Could you check a few things on this drawing? It's one solid part, dimensions in mm from its lowest x, y, z. Round coordinates to 2 decimals unless told otherwise and drop trailing zeros. Order: outer loops, then holes, each group sorted by start corner. A loop starts at its lowest first (then second) coordinate and runs counter-clockwise, first axis right, second up. Notation, with made-up numbers: (49.25, 44.25) - (94.25, 44.25) arc R26 ccw to (94.25, 70.25) - close; hole circle Ø9 at (-9, 69). An arc over 180 degrees is marked (long way). Use one line per item in the form item = value.
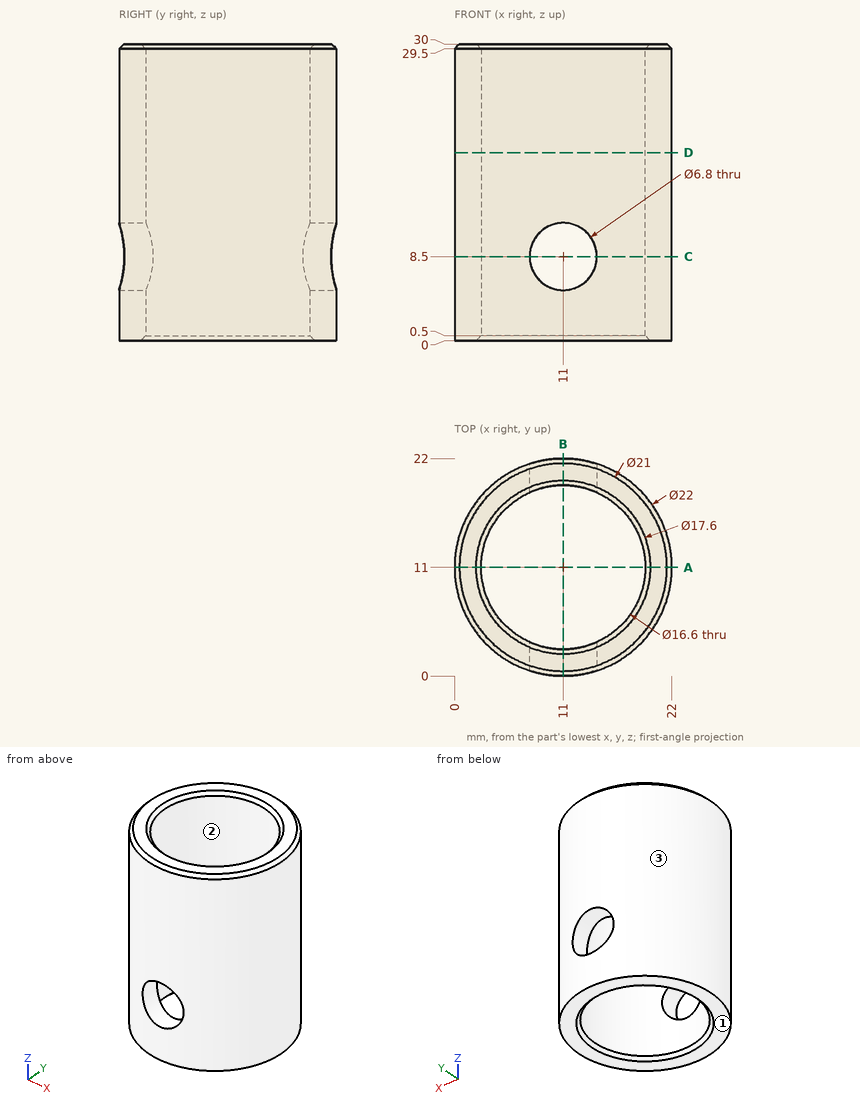
Item 1: I need wall thicknesses on L1, parallel to X at y = 10.75, z = 10; L2, parallel to Z at x = 9.25, y = 19.75. Which ranges of each line are inside material? Lowest first, please.
Found:
L1 = 0 to 2.7, 19.3 to 22
L2 = 0 to 5.58, 11.42 to 30
Item 2: Will these pins go through, and if not, where does the flat tip stop? P1, Ø12, axis at x = 17, y = 13, coming from the +Z side; P2, Ø5.5, axis at x = 11, z = 8.5, coming from the +Y side; P3, Ø1, axis at x = 3.5, z = 9, coming from the -Y side; P4, Ø6, axis at y = 3, z = 14.5, coming from the +X side.
Found:
P1 = 30
P2 = through
P3 = 2.51
P4 = 20.8
Item 3: Imagine slicing it at B-B on x = 11. Please give me the cut outline in (y, z).
Found:
outline = (0, 0) - (2.2, 0) - (2.7, 0.5) - (2.7, 5.1) - (0, 5.1) - close; (0, 11.9) - (2.7, 11.9) - (2.7, 29.5) - (2.2, 30) - (0.5, 30) - (0, 29.5) - close; (19.3, 0.5) - (19.8, 0) - (22, 0) - (22, 5.1) - (19.3, 5.1) - close; (19.3, 11.9) - (22, 11.9) - (22, 29.5) - (21.5, 30) - (19.8, 30) - (19.3, 29.5) - close
Item 4: If we mould it in two halves opening along Y, with no side actions, what happens to the marked faces 1, 2 and 3? For each: released by +Y, released by -Y, zero draft, split by the parting line, or undercut.
Found:
face_1 = zero draft
face_2 = undercut
face_3 = split by the parting line
Item 5: Imagine slicing it at D-D on z = 19. Please give me the cut outline in (x, y), plus the area to 3 significant figures.
Found:
outline = circle Ø22 at (11, 11); hole circle Ø16.6 at (11, 11)
area = 164 mm2
Item 6: Imagine slicing it at C-C on z = 8.5. Please give me the cut outline in (x, y).
Found:
outline = (7.6, 0.54) - (7.6, 3.43) arc R8.3 cw to (7.6, 18.57) - (7.6, 21.46) arc R11 ccw to start; (14.4, 0.54) arc R11 ccw to (14.4, 21.46) - (14.4, 18.57) arc R8.3 cw to (14.4, 3.43) - close
Item 7: Imagine slicing it at A-A on y = 11. Please give me the cut outline in (x, z), plus the area to 3 significant figures.
Found:
outline = (0, 0) - (2.2, 0) - (2.7, 0.5) - (2.7, 29.5) - (2.2, 30) - (0.5, 30) - (0, 29.5) - close; (19.3, 0.5) - (19.8, 0) - (22, 0) - (22, 29.5) - (21.5, 30) - (19.8, 30) - (19.3, 29.5) - close
area = 161 mm2
